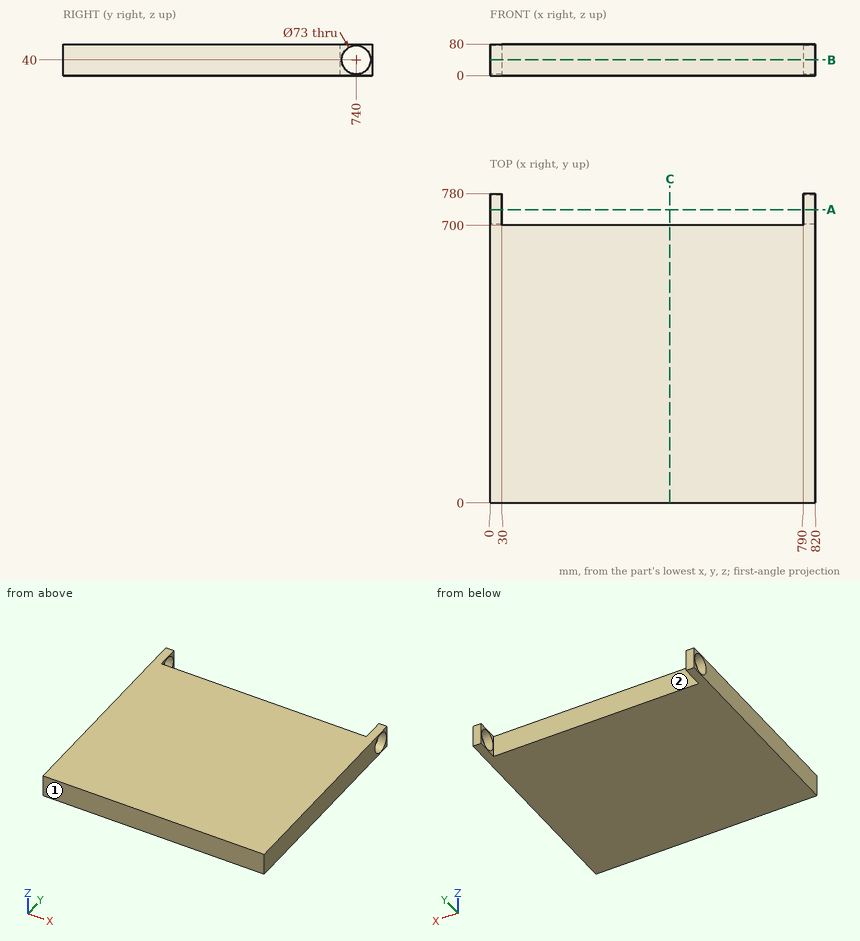
Job drawing, mm, ordinate dimensions from the low corner. One solid piece. Round coordinates to 2 decimals unless told otherwise and drop trailing zeros. Write each loop counter-clockwise with the first axis right and the second up, starting at its lowest first coordinate (ties: lowest second). Pieces come first, ordered by that corner, then holes. Notation, with made-up numbers: M 9.5,11 L 39.5,11 A16 cw 39.5,16 Z; hole C -34,55 d9. An arc over 180 degrees is marked long. Return JSON: item names as keys, results as strings. Group by question number.
(1) Saw through at C-C on x = 453.5. Write the cut outline in (y, z), then the cut area to 3 significant figures.
(2) Two-plate mould, pull along X, no slides. Class the marked faces 1 and 2: +X half, -X half, draft (parallel to the pull), parting line (faces both ways), or undercut.
(3) Saw through at B-B on z = 40. Write the cut outline in (x, y), then the cut area to 3 significant figures.
(4) Saw through at A-A on y = 740. Write the cut outline in (x, z), then the cut area to 3 significant figures.
(5) Drill centre lines: probe 1 along Y at (x, z) = (16.5, 40); probe 2 along X at (y, z) = (709, 15.5); probe 3 along Y at (x, z) = (642, 10). Where is each one in solid material? Low to high.
(6) Pin check, flat tips, straight feed: pin 1 Ø8 at (y, z) = (200.5, 56.5) entering from -X; pin 2 Ø24 at (x, z) = (515.5, 53) entering from +Y. Stop position of each tip, or through.
Returned:
{
 "1": {"outline": "M 0,0 L 700,0 L 700,80 L 0,80 Z", "area": "56,000 mm²"},
 "2": {"face 1": "draft", "face 2": "undercut"},
 "3": {"outline": "M 0,0 L 820,0 L 820,703.5 L 790,703.5 L 790,700 L 30,700 L 30,703.5 L 0,703.5 Z; M 0,776.5 L 30,776.5 L 30,780 L 0,780 Z; M 790,776.5 L 820,776.5 L 820,780 L 790,780 Z", "area": "574,000 mm²"},
 "4": {"outline": "M 0,0 L 30,0 L 30,3.5 L 0,3.5 Z; M 0,76.5 L 30,76.5 L 30,80 L 0,80 Z; M 790,0 L 820,0 L 820,3.5 L 790,3.5 Z; M 790,76.5 L 820,76.5 L 820,80 L 790,80 Z", "area": "420 mm²"},
 "5": {"probe 1": "0 to 703.5, 776.5 to 780", "probe 2": "0 to 30, 790 to 820", "probe 3": "0 to 700"},
 "6": {"pin 1": "x = 0", "pin 2": "y = 700"}
}
